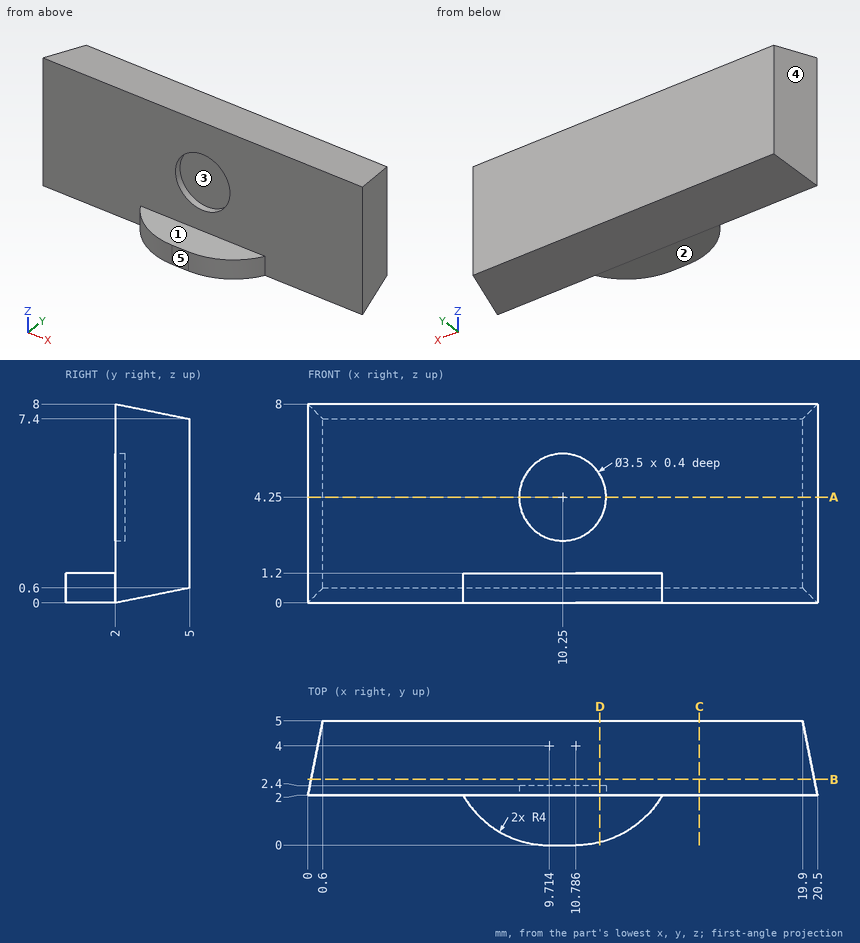
Could you check a few things on this drawing? It's one solid part, dimensions in mm from its lowest x, y, z. A direction names the side the tool comes from. Give positions to 0.01 mm unless a question says otherwise; leave off trailing zeros. Write each loop counter-clockwise with the first axis right and the second up, starting at its lowest first coordinate (ties: lowest second). Pieces come first, ordered by that corner, then holes.
(1) Will these pins go through, and if not, where does the flat tip stop? pin 1 (2 mm diameter, centred on y = 2.5, z = 6.5, fed in from -X); pin 2 (1.8 mm diameter, centred on x = 10.5, z = 4.5, fed in from -Y); pin 3 (1 mm diameter, centred on y = 1, z = 6, fed in from +X); pin 4 (2.5 mm diameter, centred on x = 9, z = 4.5, fed in from -Y).
Output values:
pin 1: stops at x = 0
pin 2: stops at y = 2.4
pin 3: passes through
pin 4: stops at y = 2
(2) Thinking about a two-plate mould opening in X: for the marked faces 3, 4 and 5, which applies, pulls with the +X half, pulls with the -X half, needs draft (parallel to the pull), parting line crosses it, or undercut?
Output values:
face 3: undercut
face 4: pulls with the -X half
face 5: needs draft
(3) Imagine slicing it at A-A, the plane z = 4.25. Write out the boundary of the cut face in (x, y), and give its area (3 significant figures).
Output values:
outline: (0, 2) - (8.5, 2) - (8.5, 2.4) - (12, 2.4) - (12, 2) - (20.5, 2) - (19.9, 5) - (0.6, 5) - close
area: 58.3 mm2
(4) Imagine slicing it at D-D, the plane x = 11.75. Write out the boundary of the cut face in (y, z).
Output values:
outline: (0.12, 0) - (2, 0) - (5, 0.6) - (5, 7.4) - (2, 8) - (2, 5.15) - (2.4, 5.15) - (2.4, 3.35) - (2, 3.35) - (2, 1.2) - (0.12, 1.2) - close
(5) Imagine slicing it at B-B, the plane y = 2.65. Write out the boundary of the cut face in (x, z).
Output values:
outline: (0.13, 0.13) - (20.37, 0.13) - (20.37, 7.87) - (0.13, 7.87) - close
(6) If I drill on L1, parallel to Y at x = 19.75, z = 7.25; L2, parallel to Z at x = 13, y = 1.6; L3, parallel to X at y = 2.2, z = 4.25, over which ranges is the centre line in solid material (lowest first)?
Output values:
L1: y = 2 to 5
L2: z = 0 to 1.2
L3: x = 0.04 to 8.5, 12 to 20.46
(7) On a 3-axis mill with a long thin cutter (end or side, diameter ignored), from which of +Z, -Z, +X, -X, +Y, -Y can I reach the whole of each face in a straight line? I mean the marked faces 1 and 2. Say none if no direction works.
Output values:
face 1: +Z, +X, -X, -Y
face 2: -Z, +X, -X, +Y, -Y
(8) Imagine slicing it at C-C, the plane x = 15.75. Write out the boundary of the cut face in (y, z).
Output values:
outline: (2, 0) - (5, 0.6) - (5, 7.4) - (2, 8) - close
